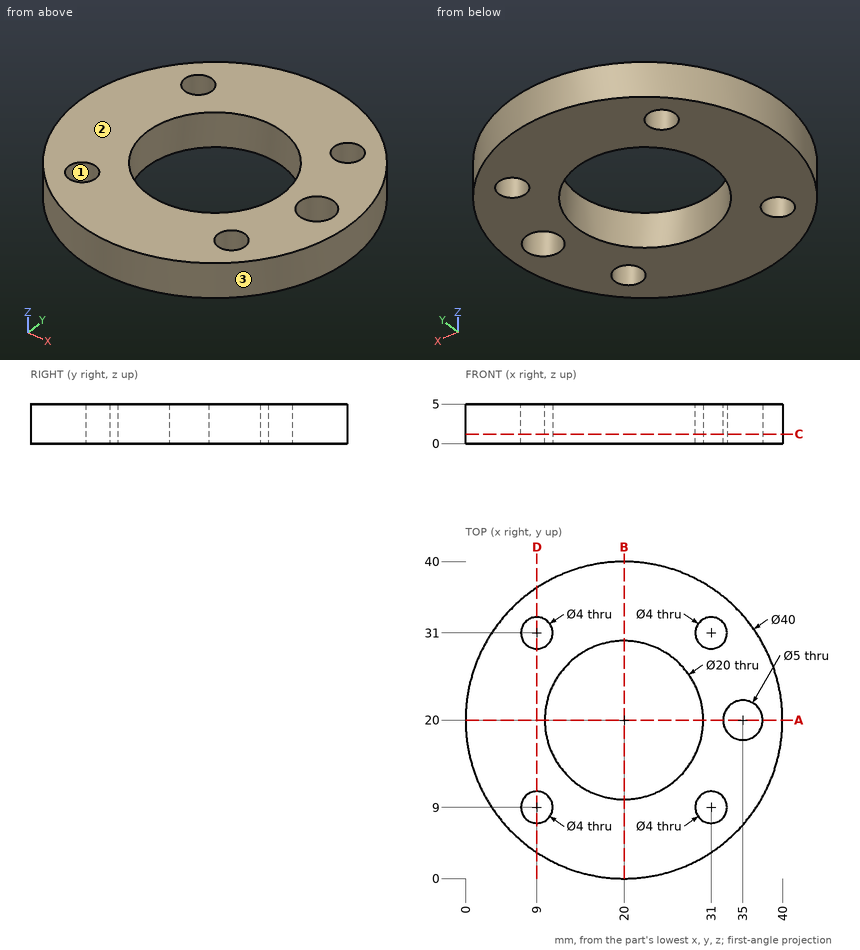
Geometry check sheet. Reference: drawing and pictorial views, mm from the part's lowest x, y, z. Round coordinates to 2 decimals unless told otherwise and drop trailing zeros. Loops run counter-clockwise (first coordinate to the right, second up) from the corner with the lowest first, then second, coordinate; pieces in that order, holes last. Notation, with made-up numbers: (-8, 80.5) - (49, 80.5) arc R31 ccw to (49, 105.5) - close; hole circle Ø4 at (43, -26.5). An arc over 180 degrees is marked (long way). Answer in a Markdown table with one row per item. Add a question column.
Q1. Section check C-C on z = 1.2. Enter the section's corners in (x, y).
Q2. Section check B-B on x = 20. Enter the section's corners in (y, z).
Q3. Section check A-A on y = 20. Enter the section's corners in (x, z).
Q4. Section check D-D on x = 9. Enter the section's corners in (y, z), plus the area to 3 significant figures.
Q5. Release check for a two-part mould opening along X. For the marked faces 1, 2 and 3 record: pulls with the +X half, pulls with the -X half, needs draft (parallel to the pull), parting line crosses it, or undercut.
Q6. Gauge pin test, flat ends, axial feed: pin 1 (6.5 mm diameter, centred on x = 31, y = 9, fed in from +Z); pin 2 (2 mm diameter, centred on x = 24.5, z = 2, fed in from -Y). Record the tip position at first contact, or that the pin passes through.
Q7. Material ranges on line 1 (X direction, y = 20, z = 1.4); line 2 (Y direction, x = 31, z = 1.65); line 3 (X direction, y = 31.5, z = 2.3), recorded low to high.
Found:
| question | item | result |
|---|---|---|
| 1 | outline | circle Ø40 at (20, 20); hole circle Ø4 at (9, 9); hole circle Ø4 at (9, 31); hole circle Ø20 at (20, 20); hole circle Ø4 at (31, 9); hole circle Ø4 at (31, 31); hole circle Ø5 at (35, 20) |
| 2 | outline | (0, 0) - (10, 0) - (10, 5) - (0, 5) - close; (30, 0) - (40, 0) - (40, 5) - (30, 5) - close |
| 3 | outline | (0, 0) - (10, 0) - (10, 5) - (0, 5) - close; (30, 0) - (32.5, 0) - (32.5, 5) - (30, 5) - close; (37.5, 0) - (40, 0) - (40, 5) - (37.5, 5) - close |
| 4 | outline | (3.3, 0) - (7, 0) - (7, 5) - (3.3, 5) - close; (11, 0) - (29, 0) - (29, 5) - (11, 5) - close; (33, 0) - (36.7, 0) - (36.7, 5) - (33, 5) - close |
| 4 | area | 127 mm² |
| 5 | face 1 | undercut |
| 5 | face 2 | needs draft |
| 5 | face 3 | parting line crosses it |
| 6 | pin 1 | stops at z = 5 |
| 6 | pin 2 | stops at y = 0.31 |
| 7 | line 1 | x = 0 to 10, 30 to 32.5, 37.5 to 40 |
| 7 | line 2 | y = 3.3 to 7, 11 to 29, 33 to 36.7 |
| 7 | line 3 | x = 3.64 to 7.06, 10.94 to 29.06, 32.94 to 36.36 |
